Autodesk Inventor part; units mm, degrees
ref_plane "YZ Plane" through (0, 0, 0) normal (1, 0, 0) x (0, 1, 0)
ref_plane "XZ Plane" through (0, 0, 0) normal (0, 1, 0) x (-1, 0, 0)
ref_plane "XY Plane" through (0, 0, 0) normal (0, 0, 1) x (1, 0, 0)
sketch "Sketch1" plane through (0, 0, 0) normal (0, 1, 0) x (-1, 0, 0)
  line L0 (3, 0) -> (54.2, 0)
  line L1 (56.2, -2) -> (56.2, -53.2)
  line L2 (53.2, -56.2) -> (3, -56.2)
  line L3 (0, -53.2) -> (0, -3)
  line L4 (56.2, 0) -> (51.7, 0)
  line L5 (51.7, 0) -> (51.7, -4.5)
  line L6 (51.7, -4.5) -> (56.2, -4.5)
  line L7 (56.2, -4.5) -> (56.2, 0)
  circle A0 centre (51.7, -4.5) radius 2.5
  line L8 (56.2, -56.2) -> (51.7, -56.2)
  line L9 (51.7, -56.2) -> (51.7, -51.7)
  line L10 (51.7, -51.7) -> (56.2, -51.7)
  line L11 (56.2, -51.7) -> (56.2, -56.2)
  circle A1 centre (51.7, -51.7) radius 2.5
  line L12 (0, 0) -> (4.5, 0)
  line L13 (4.5, 0) -> (4.5, -4.5)
  line L14 (4.5, -4.5) -> (0, -4.5)
  line L15 (0, -4.5) -> (0, 0)
  circle A2 centre (4.5, -4.5) radius 2.5
  circle A3 centre (4.5, -51.7) radius 2.5
  arc A4 (56.2, -2) -> (54.2, 0) centre (54.2, -2) ccw
  arc A5 (53.2, -56.2) -> (56.2, -53.2) centre (53.2, -53.2) ccw
  arc A6 (0, -53.2) -> (3, -56.2) centre (3, -53.2) ccw
  arc A7 (3, 0) -> (0, -3) centre (3, -3) ccw
  line L16 (51.7, -4.5) -> (4.5, -51.7)
  line L17 (4.5, -4.5) -> (51.7, -51.7)
  circle A8 centre (28.1, -28.1) radius 19
  point P0 (0, -56.2)
  dimension "d0" = 56.2
  dimension "d1" = 56.2
  dimension "d2" = 4.5
  dimension "d3" = 4.5
  dimension "d4" = 5
  dimension "d5" = 4.5
  dimension "d6" = 4.5
  dimension "d7" = 2
  dimension "d8" = 3
  dimension "d9" = 38
  dimension "d34" = 4.5
  dimension "d35" = 4.5
extrude "Extrusion1" add sketch "Sketch1" along normal blind 5 contours L0 L13 A2 L14 L3 A7 | L0 L5 A0 L16 A8 L17 A2 L13 | L0 A4 L1 L6 A0 L5 | L14 A2 L17 A8 A1 L9 L2 A6 L3 | L6 L1 L10 A1 L17 A8 L16 A0 | A8 L17 L16 | L16 L17 A8 | L17 L16 A8 | L9 A1 L10 L1 A5 L2 | L17 A8 L16
sketch "Sketch2" plane through (0, 5, 0) normal (0, 1, 0) x (1, 0, 0)
  circle A0 centre (-51.7, 4.5) radius 2.5
  circle A1 centre (-4.5, 4.5) radius 2.5
  circle A2 centre (-4.5, 51.7) radius 2.5
  circle A3 centre (-51.7, 51.7) radius 2.5
  circle A4 centre (-51.7, 4.5) radius 2.5
  line L0 (-4.5, 51.7) -> (-4.5, 4.5)
  circle A5 centre (-27.7983, 28.3967) radius 19
  line L1 (-4.5, 4.5) -> (-14.6658, 14.6658)
  line L2 (-41.5292, 41.5292) -> (-51.7, 51.7)
  line L3 (-51.7, 4.5) -> (-28.25, 27.95)
  line L4 (-14.3658, 41.8342) -> (-4.5, 51.7)
  point P0 (0, 0)
  dimension "d12" = 38
extrude "Extrusion2" add sketch "Sketch2" along normal blind 1 contours A5
sketch "Sketch3" plane through (-27.7983, 6, -28.3967) normal (0, 1, 0) x (1, 0, 0)
  circle A0 centre (0, 0) radius 3.2
  circle A1 centre (0, 0) radius 3.05
  line L0 (-3.05, 0) -> (-3.05, 0.9682)
  line L1 (-3.05, 0) -> (-3.05, -0.9682)
  point P0 (27.7983, -28.3967)
  dimension "d16" = 6.1
  dimension "d15" = 6.4
extrude "Extrusion3" add sketch "Sketch3" along normal blind 20 contours A1 | A0 L1 L0 picked at (-2.904, -1.0385)
sketch "Sketch4" plane through (0, 0, 0) normal (0, -1, 0) x (1, 0, 0)
  line L0 (-3, -56.2) -> (-53.2, -56.2)
  line L1 (-56.2, -53.2) -> (-56.2, -2)
  line L2 (-54.2, 0) -> (-3, 0)
  line L3 (0, -3) -> (0, -53.2)
  arc A0 (-56.2, -53.2) -> (-53.2, -56.2) centre (-53.2, -53.2) ccw
  line L4 (-56.2, -2) -> (-56.2, 0)
  arc A1 (-54.2, 0) -> (-56.2, -2) centre (-54.2, -2) ccw
  line L5 (-56.2, 0) -> (-54.2, 0)
  line L6 (-3, 0) -> (0, 0)
  arc A2 (0, -3) -> (-3, 0) centre (-3, -3) ccw
  line L7 (0, 0) -> (0, -3)
  arc A3 (-3, -56.2) -> (0, -53.2) centre (-3, -53.2) ccw
  line L8 (-3, -56.2) -> (0, -56.2)
  line L9 (0, -56.2) -> (0, -53.2)
  circle A4 centre (-51.7, -51.7) radius 2.5
  line L10 (-53.2, -56.2) -> (-47.2, -56.2)
  line L11 (-47.2, -55.2) -> (-47.2, -50.2)
  line L12 (-50.2, -47.2) -> (-55.2, -47.2)
  line L13 (-56.2, -47.2) -> (-56.2, -53.2)
  line L14 (-56.2, -56.2) -> (-47.2, -47.2) construction
  line L15 (-47.2, -56.2) -> (-56.2, -47.2) construction
  arc A5 (-47.2, -50.2) -> (-50.2, -47.2) centre (-50.2, -50.2) ccw
  arc A6 (-56.2, -53.2) -> (-53.2, -56.2) centre (-53.2, -53.2) ccw
  circle A7 centre (-51.7, -4.5) radius 2.5
  circle A8 centre (-4.5, -4.5) radius 2.5
  circle A9 centre (-4.5, -51.7) radius 2.5
  line L16 (-55.2, -9) -> (-50.2, -9)
  line L17 (-47.2, -6) -> (-47.2, -1)
  line L18 (-47.2, 0) -> (-56.2, 0)
  line L19 (-56.2, 0) -> (-56.2, -9)
  circle A10 centre (-51.7, -4.5) radius 2.5
  line L20 (-56.2, -9) -> (-47.2, 0) construction
  line L21 (-47.2, -9) -> (-56.2, 0) construction
  line L22 (-6, -9) -> (-1, -9)
  line L23 (0, -9) -> (0, 0)
  line L24 (0, 0) -> (-9, 0)
  line L25 (-9, -1) -> (-9, -6)
  line L26 (-9, -9) -> (0, 0) construction
  line L27 (0, -9) -> (-9, 0) construction
  line L28 (-9, -56.2) -> (0, -56.2)
  line L29 (0, -56.2) -> (0, -47.2)
  line L30 (-1, -47.2) -> (-6, -47.2)
  line L31 (-9, -50.2) -> (-9, -55.2)
  line L32 (-9, -56.2) -> (0, -47.2) construction
  line L33 (0, -56.2) -> (-9, -47.2) construction
  arc A11 (-50.2, -9) -> (-47.2, -6) centre (-50.2, -6) ccw
  arc A12 (-9, -6) -> (-6, -9) centre (-6, -6) ccw
  arc A13 (-6, -47.2) -> (-9, -50.2) centre (-6, -50.2) ccw
  line L34 (-46.2, -56.2) -> (-10, -56.2)
  line L35 (-3, -56.2) -> (-53.2, -56.2)
  line L36 (-56.2, -46.2) -> (-56.2, -10)
  line L37 (-54.2, 0) -> (-3, 0)
  line L38 (-46.2, 0) -> (-10, 0)
  line L39 (0, -10) -> (0, -46.2)
  arc A14 (-56.2, -46.2) -> (-55.2, -47.2) centre (-55.2, -46.2) ccw
  arc A15 (-47.2, -55.2) -> (-46.2, -56.2) centre (-46.2, -55.2) ccw
  arc A16 (-55.2, -9) -> (-56.2, -10) centre (-55.2, -10) ccw
  arc A17 (-46.2, 0) -> (-47.2, -1) centre (-46.2, -1) ccw
  arc A18 (-9, -1) -> (-10, 0) centre (-10, -1) ccw
  arc A19 (0, -10) -> (-1, -9) centre (-1, -10) ccw
  arc A20 (-1, -47.2) -> (0, -46.2) centre (-1, -46.2) ccw
  arc A21 (-10, -56.2) -> (-9, -55.2) centre (-10, -55.2) ccw
  point P0 (-56.2, -47.2)
  point P1 (-46.9, -55.9)
  point P2 (-9, -55.9)
  point P3 (-46.9, 0)
  point P4 (-55.9, -9)
  point P5 (-55.9, -46.9)
  point P6 (0, -46.2)
  point P7 (-56.2, -10)
  point P8 (-46.2, 0)
  point P9 (-56.2, -46.2)
  dimension "d19" = 9
  dimension "d20" = 9
  dimension "d21" = 3
  dimension "d22" = 9
  dimension "d23" = 9
  dimension "d24" = 3
  dimension "d27" = 1
extrude "Extrusion4" add sketch "Sketch4" along normal blind 80 contours L0 A15 L11 A5 L12 A14 L1 A16 L16 A11 L17 A17 L2 A18 L25 A12 L22 A19 L3 A20 L30 A13 L31 A21
sketch "Sketch5" plane through (-56.2, 0, -2) normal (-1, 0, 0) x (0, 0, 1)
  line L0 (-44.2, 0) -> (-44.2, -80)
  line L1 (-44.2, -80) -> (-26.1, -80)
  line L2 (-8, -80) -> (-44.2, -80)
  line L3 (-26.1, -80) -> (-26.1, -75)
  line L4 (-20.1, -80) -> (-32.1, -80)
  line L5 (-32.1, -80) -> (-32.1, -70)
  line L6 (-32.1, -70) -> (-20.1, -70)
  line L7 (-20.1, -70) -> (-20.1, -80)
  line L8 (-20.1, -80) -> (-32.1, -70) construction
  line L9 (-32.1, -80) -> (-20.1, -70) construction
  point P0 (2, 0)
  dimension "d28" = 18.1
  dimension "d29" = 5
  dimension "d30" = 12
  dimension "d31" = 10
extrude "Extrusion5" add sketch "Sketch5" along normal blind 1
sketch "Sketch6" plane through (0, 5, 0) normal (0, 1, 0) x (1, 0, 0)
  circle A0 centre (-27.7983, 28.3967) radius 19
  arc A1 (-53.2, 56.2) -> (-56.2, 53.2) centre (-53.2, 53.2) ccw
  line L0 (-56.2, 53.2) -> (-56.2, 2)
  arc A2 (-56.2, 2) -> (-54.2, 0) centre (-54.2, 2) ccw
  line L1 (-54.2, 0) -> (-3, 0)
  arc A3 (-3, 0) -> (0, 3) centre (-3, 3) ccw
  line L2 (0, 3) -> (0, 53.2)
  arc A4 (0, 53.2) -> (-3, 56.2) centre (-3, 53.2) ccw
  line L3 (-3, 56.2) -> (-53.2, 56.2)
  circle A5 centre (-4.5, 51.7) radius 2.5
  circle A6 centre (-51.7, 51.7) radius 2.5
  circle A7 centre (-4.5, 4.5) radius 2.5
  circle A8 centre (-51.7, 4.5) radius 2.5
  point P0 (0, 0)
sketch "Sketch7" plane through (-54.2, 5, 0) normal (0, 0, 1) x (1, 0, 0)
  line L0 (44.2, -85) -> (8, -85)
  line L1 (26.1, -85) -> (26.1, -82)
  circle A0 centre (26.1, -82) radius 3
  point P0 (54.2, -5)
  dimension "d36" = 3
sketch "Sketch8" plane through (0, 0, -53.2) normal (1, 0, 0) x (0, 0, -1)
  line L0 (-7, -80) -> (-43.2, -80)
  line L1 (-25.1, -80) -> (-25.1, -77)
  circle A0 centre (-25.1, -77) radius 3
  point P0 (-53.2, 0)
  dimension "d37" = 3
equation "\"BendRadius\" = Thickness"
equation "\"BendReliefWidth\" = Thickness"
equation "\"BendReliefDepth\" = 0.5 * Thickness"
equation "\"CornerReliefSize\" = 4 * Thickness"
equation "\"MinimumRemnant\" = 2 * Thickness"
equation "\"TransitionRadius\" = BendRadius"
equation "\"JacobiRadiusSize\" = BendRadius"
equation "\"GapSize\" = Thickness"
properties part number "motor"
Input: part model. Units: mm. Frame: model coordinates. A direction names the side the tool comes from. Give positions to 0.01 mm unless a question says otherwise; leave off trailing zeros. Loops run counter-clockwise (first coordinate to the right, second up) from the corner with the lowest first, then second, coordinate; pieces in that order, holes last. Notation, with made-up numbers: M -20,35 L 13,35 A21 ccw 13,61 Z; hole C 7,57 d2. An arc over 180 degrees is marked long. Answer as CSV lines item,"result". Start each with the question number.
1. Pin query (flat end, axial travel): P1, Ø8, axis at x = -9.5, y = -38.5, coming from the -Z side; P2, Ø5.5, axis at y = -36.5, z = -3, coming from the +X side; P3, Ø4.5, axis at x = -51.7, z = -4.5, coming from the +Y side; P4, Ø3, axis at y = -63, z = -30, coming from the -X side. Return the tip coordinate at first contact, or that it passes through.
2. Line query: L1, parallel to X at y = 2.55, z = -4.5; L2, parallel to Z at x = -4, y = 2. Output: solid intervals per line, ascending.
3. Section A-A on z = -51.7. Return loops of the section in (x, y), plus the area to 3 significant figures.
4. Reachability of faces 1 (the face through (-48.1, -39.44, -48.06)), 2 (the face through (-1.6, 0, -3.8)), 3 (the face through (-53, -39, -9)), 4 (the face through (-4, 0, -49)) from +Z, -Z, +X, -X, +Y, -Y: full face, straight path, thin tool, end or side. Return the list, or none.
5. Section D-D on x = -20. Return loops of the section in (y, z).
6. Section C-C on y = -41. Return loops of the section in (x, z).
7. Section B-B on x = -4.5. Return loops of the section in (y, z).
Computed values:
1,P1,"stops at z = -56.2"
1,P2,"stops at x = -9"
1,P3,"passes through"
1,P4,"stops at x = -56.2"
2,L1,"x = -56.2 to -54.2, -49.2 to -7, -2 to 0"
2,L2,"z = -56.2 to -54.15, -49.25 to -6.95, -2.05 to 0"
3,outline,"M -56.2,0 L -54.2,0 L -54.2,5 L -56.2,5 Z; M -49.2,0 L -47.2,0 L -47.2,-80 L -9,-80 L -9,0 L -7,0 L -7,5 L -49.2,5 Z; M -2,0 L 0,0 L 0,5 L -2,5 Z"
3,area,"3,290 mm²"
4,face 1,"-Z, -X, -Y"
4,face 2,"+Z, +X, -Y"
4,face 3,"+Z, -X, -Y"
4,face 4,"-Z, +X, -Y"
5,outline,"M -80,-56.2 L 5,-56.2 L 5,-45.72 L 6,-45.72 L 6,-11.07 L 5,-11.07 L 5,0 L -80,0 Z"
6,outline,"M -56.2,-46.2 A1 ccw -55.2,-47.2 L -50.2,-47.2 A3 cw -47.2,-50.2 L -47.2,-55.2 A1 ccw -46.2,-56.2 L -10,-56.2 A1 ccw -9,-55.2 L -9,-50.2 A3 cw -6,-47.2 L -1,-47.2 A1 ccw 0,-46.2 L 0,-10 A1 ccw -1,-9 L -6,-9 A3 cw -9,-6 L -9,-1 A1 ccw -10,0 L -46.2,0 A1 ccw -47.2,-1 L -47.2,-6 A3 cw -50.2,-9 L -55.2,-9 A1 ccw -56.2,-10 Z"
7,outline,"M -80,-47.2 L 0,-47.2 L 0,-49.2 L 5,-49.2 L 5,-7 L 0,-7 L 0,-9 L -80,-9 Z; M 0,-56.2 L 5,-56.2 L 5,-54.2 L 0,-54.2 Z; M 0,-2 L 5,-2 L 5,0 L 0,0 Z"
